```python
from build123d import *

# Parameters (mm, degrees)
SKETCH1_W                = 100
SKETCH1_H                = 40
BOSS_EXTRUDE1_DEPTH      = 4
FILLET1_R                = 2
M5_CLEARANCE_HOLE1_D     = 5.3
M5_CLEARANCE_HOLE1_DEPTH = 8
M5_CLEARANCE_HOLE1_TIP   = 1.59228064


with BuildPart() as part:
    # Sketch1 → Boss-Extrude1 (new body)
    with BuildSketch(Plane(origin=(0, 0, 0), x_dir=(1, 0, 0), z_dir=(0, 1, 0))):
        Rectangle(SKETCH1_W, SKETCH1_H)
    extrude(amount=BOSS_EXTRUDE1_DEPTH)

    # Fillet1
    fillet1_edges = [part.edges().sort_by_distance(p)[0] for p in [
        (-50, 2, -20),
        (50, 2, -20),
        (50, 2, 20),
        (-50, 2, 20),
    ]]
    fillet(fillet1_edges, radius=FILLET1_R)

    # M5 Clearance Hole1
    with Locations(Plane(origin=(0, 4, 0), x_dir=(1, 0, 0), z_dir=(0, 1, 0))):
        with Locations((-40, 5), (-23, 5), (-23, -10), (23, -10), (23, 5), (40, 5)):
            Hole(M5_CLEARANCE_HOLE1_D / 2, depth=M5_CLEARANCE_HOLE1_DEPTH)
            with Locations((0, 0, -(M5_CLEARANCE_HOLE1_DEPTH + M5_CLEARANCE_HOLE1_TIP / 2))):  # 118° drill point
                Cone(0, M5_CLEARANCE_HOLE1_D / 2, M5_CLEARANCE_HOLE1_TIP, mode=Mode.SUBTRACT)


solid = part.part
```
Geometry: final body of the model. Coordinates: model frame, mm. Give positions to 0.01 mm unless a question says otherwise; leave off trailing zeros. Write each loop counter-clockwise with the first axis right and the second up, starting at its lowest first coordinate (ties: lowest second). Pieces come first, ordered by that corner, then holes.
1. Draft query along Z for faces 1 (the flat face through (-1, 2, -20)), 2 (the flat face through (-1, 0, 0)), 3 (the cylindrical face through (42.647, 1.972, -5.117)). Return one class per face: released by +Z, released by -Z, zero draft, split by the parting line, or undercut.
2. Pin query (flat end, axial travel): P1, Ø7, axis at x = -23, z = -5, coming from the +Y side. Return the tip coordinate at first contact, or that it passes through.
3. Line query: probe 1 along Z at (x, y) = (23, 1.65); probe 2 along X at (y, z) = (3.05, 10); probe 3 along Z at (x, y) = (-40, 1.2). Output: solid intervals per line, ascending.
4. Section query A-A, the plane z = 10. Return loops of the section in (x, y).
5. Section query C-C, the plane y = 0.6. Return loops of the section in (x, z), then the cut area to 3 significant figures.
6. Section query B-B, the plane x = 40. Return loops of the section in (y, z), then the cut area to 3 significant figures.
7. Section query D-D, the plane z = -5. Return loops of the section in (x, y), then the cut area to 3 significant figures.
Computed:
1. face 1: released by -Z
1. face 2: zero draft
1. face 3: undercut
2. P1: stops at y = 4
3. probe 1: z = -20 to -7.65, -2.35 to 7.35, 12.65 to 20
3. probe 2: x = -50 to -25.65, -20.35 to 20.35, 25.65 to 50
3. probe 3: z = -20 to -7.65, -2.35 to 20
4. outline: (-50, 0) - (-25.65, 0) - (-25.65, 4) - (-50, 4) - close; (-20.35, 0) - (20.35, 0) - (20.35, 4) - (-20.35, 4) - close; (25.65, 0) - (50, 0) - (50, 4) - (25.65, 4) - close
5. outline: (-50, -18) arc R2 ccw to (-48, -20) - (48, -20) arc R2 ccw to (50, -18) - (50, 18) arc R2 ccw to (48, 20) - (-48, 20) arc R2 ccw to (-50, 18) - close; hole circle Ø5.3 at (-40, -5); hole circle Ø5.3 at (-23, -5); hole circle Ø5.3 at (-23, 10); hole circle Ø5.3 at (23, -5); hole circle Ø5.3 at (23, 10); hole circle Ø5.3 at (40, -5)
5. area: 3,860 mm2
6. outline: (0, -20) - (4, -20) - (4, -7.65) - (0, -7.65) - close; (0, -2.35) - (4, -2.35) - (4, 20) - (0, 20) - close
6. area: 139 mm2
7. outline: (-50, 0) - (-42.65, 0) - (-42.65, 4) - (-50, 4) - close; (-37.35, 0) - (-25.65, 0) - (-25.65, 4) - (-37.35, 4) - close; (-20.35, 0) - (20.35, 0) - (20.35, 4) - (-20.35, 4) - close; (25.65, 0) - (37.35, 0) - (37.35, 4) - (25.65, 4) - close; (42.65, 0) - (50, 0) - (50, 4) - (42.65, 4) - close
7. area: 315 mm2
